Autodesk Inventor part; units mm, degrees
ref_plane "YZ Plane" through (0, 0, 0) normal (1, 0, 0) x (0, 1, 0)
ref_plane "XZ Plane" through (0, 0, 0) normal (0, 1, 0) x (-1, 0, 0)
ref_plane "XY Plane" through (0, 0, 0) normal (0, 0, 1) x (1, 0, 0)
sketch "Sketch1" plane through (0, 0, 0) normal (0, 1, 0) x (-1, 0, 0)
  line L0 (0, 0) -> (0, 76.2)
  line L1 (25.4, 76.2) -> (25.4, 25.4)
  line L2 (25.4, 25.4) -> (76.2, 25.4)
  line L3 (76.2, 25.4) -> (76.2, 0)
  line L4 (76.2, 0) -> (0, 0)
  line L5 (25.4, 25.4) -> (0, 0) construction
  circle A0 centre (12.7, 63.5) radius 3.3782
  circle A1 centre (12.7, 25.4) radius 3.3782
  circle A2 centre (25.4, 12.7) radius 3.3782
  circle A3 centre (63.5, 12.7) radius 3.3782
  line L6 (25.4, 76.2) -> (25.4, 95.25)
  line L7 (25.4, 95.25) -> (0, 95.25)
  line L8 (0, 95.25) -> (0, 76.2)
  point P0 (0, 0)
  dimension "d0" = 76.2
  dimension "d1" = 25.4
  dimension "d2" = 50.8
  dimension "d3" = 50.8
  dimension "d4" = 25.4
  dimension "d5" = 6.7564
  dimension "d6" = 6.7564
  dimension "d7" = 6.7564
  dimension "d8" = 6.7564
  dimension "d9" = 12.7
  dimension "d10" = 0
  dimension "d11" = 12.7
  dimension "d12" = 12.7
  dimension "d13" = 12.7
  dimension "d15" = 12.7
  dimension "d17" = 19.05
extrude "Plate1" add sketch "Sketch1" along normal blind 3.175
sketch "Sketch2" plane through (0, 0, 92.075) normal (0, 0, 1) x (1, 0, 0)
  line L0 (-25.4, 0) -> (0, 0)
  line L1 (0, 0) -> (0, 76.2)
  line L2 (0, 76.2) -> (-25.4, 76.2)
  line L3 (-25.4, 76.2) -> (-25.4, 0)
edge flange "Flange1" height 76.2 angle 90 thickness 3.175 bend radius 1.27 thickness toward (0, 0, 1) relief tear relief width 3.175 relief depth 1.5875 edges at (-12.7, 3.175, 95.25) wall of the first edge with corners at (-25.4, 0, 92.075) (0, 0, 92.075) (0, 76.2, 92.075) (-25.4, 76.2, 92.075)
bend "Bend1"
corner "Corner1"
sketch "Sketch3" plane through (0, 76.2, 92.075) normal (0, 0, -1) x (-1, 0, 0)
  line L0 (25.4, 0) -> (0, 0)
  circle A0 centre (12.7, -12.7) radius 3.3782
  circle A1 centre (12.7, -63.5) radius 3.3782
  point P0 (0, -76.2)
  dimension "d29" = 6.7564
  dimension "d30" = 6.7564
  dimension "d31" = 12.7
  dimension "d32" = 50.8
extrude "Cut1" cut sketch "Sketch3" against normal blind 3.175
equation "\"d33\" = Thickness"
equation "\"d19\" = BendReliefWidth"
equation "\"d20\" = BendReliefDepth"
equation "\"d21\" = MinimumRemnant"
equation "\"d22\" = BendRadius"
equation "\"d26\" = CornerReliefSize"
equation "\"d27\" = GapSize"
equation "\"d28\" = JacobiRadiusSize"
equation "\"BendRadius\" = Thickness"
equation "\"BendReliefWidth\" = Thickness"
equation "\"BendReliefDepth\" = 0.5 * Thickness"
equation "\"CornerReliefSize\" = 4 * Thickness"
equation "\"MinimumRemnant\" = 2 * Thickness"
equation "\"TransitionRadius\" = BendRadius"
equation "\"JacobiRadiusSize\" = BendRadius"
equation "\"GapSize\" = Thickness"
equation "\"d18\" = BendRadius"
properties part number "Rebuild Gusset 2" material "Aluminum 6061"
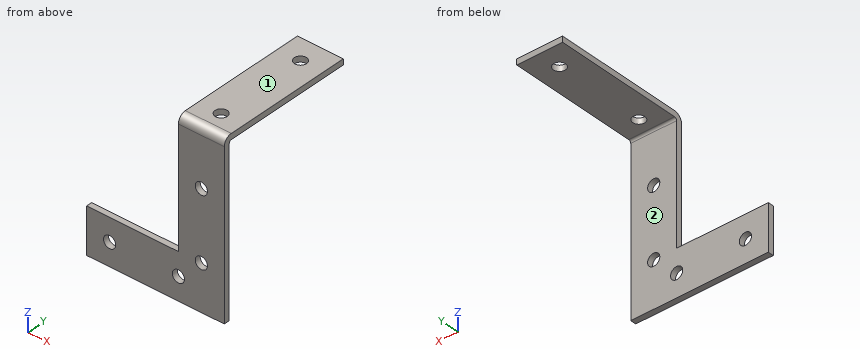
Can you work these out from the model? Positions are in its coordinate system, mm. Face numbers are marked on the shaded views. A direction names the side the tool comes from. Give positions to 0.01 mm unless a question says otherwise; leave off trailing zeros. Order: outer loops, then holes, each group sorted by start corner. A loop starts at its lowest first (then second) coordinate and runs counter-clockwise, first axis right, second up. Notation, with made-up numbers: M 75,-2 L 131,-2 A25 cw 131,33 Z; hole C 76,82.25 d10. An arc over 180 degrees is marked long. Use a Markdown table: item, result. Add a question column.
Item 1: Suppose I cut it at A-A (y = 12.7). List the corners of the cut face in (x, z) for me (3 decimals).
Item 2: Suppose I cut it at D-D (x = -12.7). List the corners of the cut face in (y, z) for me (3 decimals), then the cut area to 3 significant figures.
Item 3: If I drill on L1, parallel to X at y = 2, z = 12; L2, parallel to X at y = 1, z = 63; L3, parallel to Y at x = -25, z = 65.5 (3 decimals), over which ranges is the centre line in solid material (lowest first)? Write a range as [from, to].
Item 4: For the marked faces 1 and 2, which set-ups out of +Z, -Z, +X, -X, +Y, -Y let a thin tool reach every point of the face, with its end or its side?
Item 5: Will these pins go through, and if not, where does the flat tip stop? pin 1 (12.5 mm diameter, centred on x = -13, y = 28, fed in from -Z) (3 decimals); pin 2 (9 mm diameter, centred on x = -12.7, z = 25.4, fed in from +Y) (3 decimals); pin 3 (1 mm diameter, centred on x = -57.5, y = 1.5, fed in from +Z).
Item 6: Suppose I cut it at C-C (z = 12.7). List the corners of the cut face in (x, y) for me (3 decimals).
Item 7: Suppose I cut it at B-B (x = -63.5). List the corners of the cut face in (y, z) for me (3 decimals), then the cut area to 3 significant figures.
Answer sheet:
| question | item | result |
|---|---|---|
| 1 | outline | M -25.4,92.075 L -16.078,92.075 L -16.078,95.25 L -25.4,95.25 Z; M -9.322,92.075 L 0,92.075 L 0,95.25 L -9.322,95.25 Z |
| 2 | outline | M 0,0 L 3.175,0 L 3.175,22.022 L 0,22.022 Z; M 0,28.778 L 3.175,28.778 L 3.175,60.122 L 0,60.122 Z; M 0,66.878 L 3.175,66.878 L 3.175,90.805 A1.27 cw 4.445,92.075 L 9.322,92.075 L 9.322,95.25 L 4.445,95.25 A4.445 ccw 0,90.805 Z; M 16.078,92.075 L 60.122,92.075 L 60.122,95.25 L 16.078,95.25 Z; M 66.878,92.075 L 76.2,92.075 L 76.2,95.25 L 66.878,95.25 Z |
| 2 | area | 445 mm² |
| 3 | L1 | x = [-76.2, -66.8], [-60.2, -28.7], [-22.1, 0] |
| 3 | L2 | x = [-25.4, -16.04], [-9.36, 0] |
| 3 | L3 | y = [0, 3.175] |
| 4 | face 1 | +Z, +X, -X, +Y, -Y |
| 4 | face 2 | -Z, +X, -X, +Y |
| 5 | pin 1 | stops at z = 92.075 |
| 5 | pin 2 | stops at y = 3.175 |
| 5 | pin 3 | stops at z = 25.4 |
| 6 | outline | M -76.2,0 L -66.878,0 L -66.878,3.175 L -76.2,3.175 Z; M -60.122,0 L -28.778,0 L -28.778,3.175 L -60.122,3.175 Z; M -22.022,0 L 0,0 L 0,3.175 L -22.022,3.175 Z |
| 7 | outline | M 0,0 L 3.175,0 L 3.175,9.322 L 0,9.322 Z; M 0,16.078 L 3.175,16.078 L 3.175,25.4 L 0,25.4 Z |
| 7 | area | 59.2 mm² |
